Source: CAD feature listing. Evaluate the final solid. Frame: model axes, mm. A direction names the side the tool comes from. Round coordinates to 2 decimals unless told otherwise and drop trailing zeros. Loops run counter-clockwise (first coordinate to the right, second up) from the corner with the lowest first, then second, coordinate; pieces in that order, holes last. Notation, with made-up numbers: (-22.75, 75) -> (34.25, 75) arc R22 ccw to (34.25, 94) -> close; hole circle Ø10 at (62, 7.25). An arc over 180 degrees is marked (long way). Return JSON: item names as keys, results as strings. Group by question number.
```python
from build123d import *

# Parameters (mm, degrees)
BOSS_EXTRUDE1_DEPTH  = 10
BOSS_EXTRUDE2_DEPTH  = 5
BOSS_EXTRUDE3_DEPTH  = 60
FILLET1_R            = 5
FILLET1_OF_MIRROR1_R = 5
BOSS_EXTRUDE4_DEPTH  = 3
FILLET2_R            = 5


with BuildPart() as part:
    # Sketch1 → Boss-Extrude1 (new body)
    with BuildSketch(Plane(origin=(0, 0, 0), x_dir=(1, 0, 0), z_dir=(0, 1, 0))):
        Polygon((-5.773502692, -10), (5.773502692, -10), (11.547005384, 0), (5.773502692, 10), (-5.773502692, 10), (-11.547005384, 0), align=None)
        Polygon((-4.041451884, -7), (4.041451884, -7), (8.082903769, 0), (4.041451884, 7), (-4.041451884, 7), (-8.082903769, 0), align=None, mode=Mode.SUBTRACT)
    boss_extrude1 = extrude(amount=BOSS_EXTRUDE1_DEPTH)

    # Sketch1<3> → Boss-Extrude2 (add)
    # profile 1 of 2: a face of its own
    with BuildSketch(Plane(origin=(0, 0, 0), x_dir=(1, 0, 0), z_dir=(0, 1, 0))):
        Polygon((-6.92820323, -12), (6.92820323, -12), (13.856406461, 0), (6.92820323, 12), (-6.92820323, 12), (-13.856406461, 0), align=None)
        Polygon((5.773502692, -10), (11.547005384, 0), (5.773502692, 10), (-5.773502692, 10), (-11.547005384, 0), (-5.773502692, -10), align=None, mode=Mode.SUBTRACT)
    # profile 2 of 2: a face of its own
    with BuildSketch(Plane(origin=(0, 0, 0), x_dir=(1, 0, 0), z_dir=(0, 1, 0))):
        Polygon((-5.773502692, -10), (5.773502692, -10), (11.547005384, 0), (5.773502692, 10), (-5.773502692, 10), (-11.547005384, 0), align=None)
        Polygon((-4.041451884, -7), (4.041451884, -7), (8.082903769, 0), (4.041451884, 7), (-4.041451884, 7), (-8.082903769, 0), align=None, mode=Mode.SUBTRACT)
    boss_extrude2 = extrude(amount=-BOSS_EXTRUDE2_DEPTH)

    # Sketch1<4> → Boss-Extrude3 (add)
    with BuildSketch(Plane(origin=(0, 0, 0), x_dir=(1, 0, 0), z_dir=(0, 1, 0))):
        Polygon((-8.660254038, -15), (8.660254038, -15), (17.320508076, 0), (8.660254038, 15), (-8.660254038, 15), (-17.320508076, 0), align=None)
        Polygon((6.92820323, -12), (13.856406461, 0), (6.92820323, 12), (-6.92820323, 12), (-13.856406461, 0), (-6.92820323, -12), align=None, mode=Mode.SUBTRACT)
    boss_extrude3 = extrude(amount=-BOSS_EXTRUDE3_DEPTH)

    # Fillet1
    fillet1_edges = [part.edges().sort_by_distance(p)[0] for p in [
        (8.660254038, -30, 15),
        (-8.660254038, -30, 15),
        (-17.320508076, -30, 0),
        (-8.660254038, -30, -15),
        (8.660254038, -30, -15),
        (17.320508076, -30, 0),
    ]]
    fillet(fillet1_edges, radius=FILLET1_R)

    # Mirror1: Boss-Extrude1, Boss-Extrude2, Boss-Extrude3 across plane
    add(boss_extrude1.mirror(Plane.ZX.offset(10)))
    add(boss_extrude2.mirror(Plane.ZX.offset(10)))
    add(boss_extrude3.mirror(Plane.ZX.offset(10)))

    # Fillet1 of Mirror1
    fillet1_of_mirror1_edges = [part.edges().sort_by_distance(p)[0] for p in [
        (8.660254038, 50, 15),
        (-8.660254038, 50, 15),
        (-17.320508076, 50, 0),
        (-8.660254038, 50, -15),
        (8.660254038, 50, -15),
        (17.320508076, 50, 0),
    ]]
    fillet(fillet1_of_mirror1_edges, radius=FILLET1_OF_MIRROR1_R)

    # Sketch2 → Boss-Extrude4 (add)
    # profile 1 of 6: a face of its own
    with BuildSketch(Plane(origin=(0, 80, 0), x_dir=(1, 0, 0), z_dir=(0, 1, 0))):
        with BuildLine():
            ThreePointArc((10.103629711, 12.5), (8.273502692, 14.330127019), (5.773502692, 15))
            Line((5.773502692, 15), (-5.773502692, 15))
            ThreePointArc((-5.773502692, 15), (-8.273502692, 14.330127019), (-10.103629711, 12.5))
            Line((-10.103629711, 12.5), (-15.877132403, 2.5))
            ThreePointArc((-15.877132403, 2.5), (-16.547005384, 0), (-15.877132403, -2.5))
            Line((-15.877132403, -2.5), (-10.103629711, -12.5))
            ThreePointArc((-10.103629711, -12.5), (-8.273502692, -14.330127019), (-5.773502692, -15))
            Line((-5.773502692, -15), (5.773502692, -15))
            ThreePointArc((5.773502692, -15), (8.273502692, -14.330127019), (10.103629711, -12.5))
            Line((10.103629711, -12.5), (15.877132403, -2.5))
            ThreePointArc((15.877132403, -2.5), (16.547005384, 0), (15.877132403, 2.5))
            Line((15.877132403, 2.5), (10.103629711, 12.5))
        make_face()
        Polygon((6.92820323, 12), (13.856406461, 0), (6.92820323, -12), (-6.92820323, -12), (-13.856406461, 0), (-6.92820323, 12), align=None, mode=Mode.SUBTRACT)
    # profile 2 of 6: a face of its own
    with BuildSketch(Plane(origin=(0, 80, 0), x_dir=(1, 0, 0), z_dir=(0, 1, 0))):
        Polygon((-6.92820323, 12), (-12.413030788, 2.5), (12.413030788, 2.5), (6.92820323, 12), align=None)
    # profile 3 of 6: a face of its own
    with BuildSketch(Plane(origin=(0, 80, 0), x_dir=(1, 0, 0), z_dir=(0, 1, 0))):
        Polygon((12.413030788, -2.5), (-12.413030788, -2.5), (-6.92820323, -12), (6.92820323, -12), align=None)
    # profile 4 of 6: a face of its own
    with BuildSketch(Plane(origin=(0, 80, 0), x_dir=(1, 0, 0), z_dir=(0, 1, 0))):
        with BuildLine():
            Line((-12.413030788, -2.5), (-15.877132403, -2.5))
            Line((-15.877132403, -2.5), (-10.103629711, -12.5))
            ThreePointArc((-10.103629711, -12.5), (-8.273502692, -14.330127019), (-5.773502692, -15))
            Line((-5.773502692, -15), (5.773502692, -15))
            ThreePointArc((5.773502692, -15), (8.273502692, -14.330127019), (10.103629711, -12.5))
            Line((10.103629711, -12.5), (15.877132403, -2.5))
            Line((15.877132403, -2.5), (12.413030788, -2.5))
            Line((12.413030788, -2.5), (6.92820323, -12))
            Line((6.92820323, -12), (-6.92820323, -12))
            Line((-6.92820323, -12), (-12.413030788, -2.5))
        make_face()
    # profile 5 of 6: a face of its own
    with BuildSketch(Plane(origin=(0, 80, 0), x_dir=(1, 0, 0), z_dir=(0, 1, 0))):
        with BuildLine():
            Line((15.877132403, 2.5), (12.413030788, 2.5))
            Line((12.413030788, 2.5), (13.856406461, 0))
            Line((13.856406461, 0), (12.413030788, -2.5))
            Line((12.413030788, -2.5), (15.877132403, -2.5))
            ThreePointArc((15.877132403, -2.5), (16.547005384, 0), (15.877132403, 2.5))
        make_face()
    # profile 6 of 6: a face of its own
    with BuildSketch(Plane(origin=(0, 80, 0), x_dir=(1, 0, 0), z_dir=(0, 1, 0))):
        with BuildLine():
            Line((-12.413030788, 2.5), (-15.877132403, 2.5))
            ThreePointArc((-15.877132403, 2.5), (-16.547005384, 0), (-15.877132403, -2.5))
            Line((-15.877132403, -2.5), (-12.413030788, -2.5))
            Line((-12.413030788, -2.5), (-13.856406461, 0))
            Line((-13.856406461, 0), (-12.413030788, 2.5))
        make_face()
    extrude(amount=BOSS_EXTRUDE4_DEPTH)

    # Fillet2
    fillet2_edges = [part.edges().sort_by_distance(p)[0] for p in [
        (-8.660254038, 0, 5),
        (-8.660254038, 0, -5),
        (0, 0, -10),
        (8.660254038, 0, -5),
        (0, 20, 10),
        (8.660254038, 20, 5),
        (8.660254038, 20, -5),
        (0, 20, -10),
        (-8.660254038, 20, -5),
        (-8.660254038, 20, 5),
        (8.660254038, 0, 5),
        (0, 0, 10),
        (-5.773502692, 10, 10),
        (-11.547005384, 10, 0),
        (-5.773502692, 10, -10),
        (5.773502692, 10, -10),
        (11.547005384, 10, 0),
        (5.773502692, 10, 10),
    ]]
    fillet(fillet2_edges, radius=FILLET2_R - 0.0001)  # a hair under: the kernel refuses the full size


solid = part.part
```
(1) Ray query, line 1 (Z direction, x = -5, y = -49); line 2 (X direction, y = 41, z = 0); line 3 (Y direction, x = 8, z = 6). Return the intervals inside material, ascending.
(2) Set-up query: faces 5 (the face through (8.64, 10.07, 5.035)), 6 (the face through (6.034, 9.79, 3.549)), 7 (the face through (0, 80, 7)), 8 (the face through (-5.42, 9.93, 9.31)), 9 (the face through (-9.983, 18.574, -5.717)). Return all of +Z, -Z, +X, -X, +Y, -Y with unobstructed straight access to the full face (end or side cutting, diameter ignored); none if empty.
(3) Mould query, pull axis Z, two halves, no side actions, for faces 1 (the face through (0, 51, 15)), 2 (the face through (-16.547, -30.42, 0.037)), 3 (the face through (-6.09, 9.79, 3.45)), 4 (the face through (-10.44, 53.59, -5.92)). Classes: released by +Z, released by -Z, zero draft, split by the parting line, or undercut.
(4) Cut plane A-A (y = 50). Return loops of the section in (x, z).
(5) Cut plane B-B (y = 7.5). Return loops of the section in (x, z), and give its area (3 significant figures).
(6) Pin query (flat end, axial travel): pin 1 (6 mm diameter, centred on y = 50, z = -5.5, fed in from -X); pin 2 (2 mm diameter, centred on y = -32, z = -2, fed in from -X); pin 3 (6.5 mm diameter, centred on x = -0.5, y = 4, fed in from +Z). Return the tip coordinate at first contact, or that it passes through.
Answers follow:
{
 "1": {"line 1": "-15 to -12, 12 to 15", "line 2": "-16.55 to -13.86, 13.86 to 16.55", "line 3": "-5 to 25, 80 to 83"},
 "2": {"face 5": "+Z, +X", "face 6": "-Y", "face 7": "none", "face 8": "+Z, -X", "face 9": "-Z, -X"},
 "3": {"face 1": "released by +Z", "face 2": "split by the parting line", "face 3": "undercut", "face 4": "undercut"},
 "4": {"outline": "(-15.88, -2.5) -> (-10.1, -12.5) arc R5 ccw to (-5.77, -15) -> (5.77, -15) arc R5 ccw to (10.1, -12.5) -> (15.88, -2.5) arc R5 ccw to (15.88, 2.5) -> (10.1, 12.5) arc R5 ccw to (5.77, 15) -> (-5.77, 15) arc R5 ccw to (-10.1, 12.5) -> (-15.88, 2.5) arc R5 ccw to start; hole (-13.86, 0) -> (-6.93, -12) -> (6.93, -12) -> (13.86, 0) -> (6.93, 12) -> (-6.93, 12) -> close"},
 "5": {"outline": "(-10.1, -2.5) -> (-7.22, -7.5) arc R5 ccw to (-2.89, -10) -> (2.89, -10) arc R5 ccw to (7.22, -7.5) -> (10.1, -2.5) arc R5 ccw to (10.1, 2.5) -> (7.22, 7.5) arc R5 ccw to (2.89, 10) -> (-2.89, 10) arc R5 ccw to (-7.22, 7.5) -> (-10.1, 2.5) arc R5 ccw to start; hole (-8.08, 0) -> (-4.04, -7) -> (4.04, -7) -> (8.08, 0) -> (4.04, 7) -> (-4.04, 7) -> close", "area": "169 mm^2"},
 "6": {"pin 1": "x = -15.88", "pin 2": "x = -16.45", "pin 3": "z = 12.37"}
}
